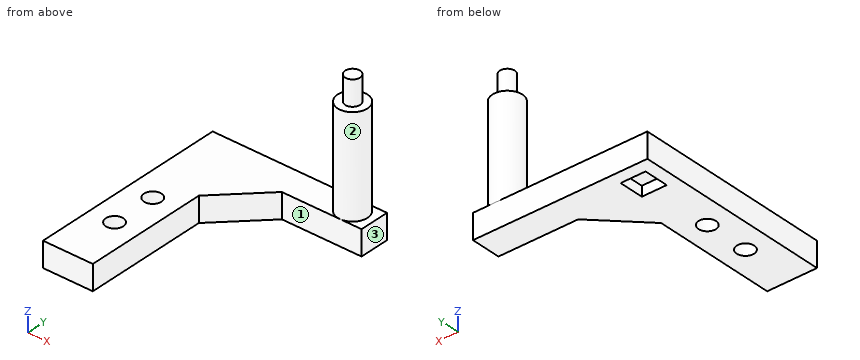
```python
from build123d import *

# Parameters (mm, degrees)
SKIZZE2_W                       = 10
SKIZZE2_H                       = 40
AUFSATZ_LINEAR_AUSTRAGEN1_DEPTH = 5
SKIZZE4_R                       = 1.75
SCHNITT_LINEAR_AUSTRAGEN1_DEPTH = 5
SKIZZE5_W                       = 5
SKIZZE5_H                       = 5
SCHNITT_LINEAR_AUSTRAGEN2_DEPTH = 2
SKIZZE6_W                       = 25
SKIZZE6_H                       = 6
AUFSATZ_LINEAR_AUSTRAGEN3_DEPTH = 5
SKIZZE7_R                       = 3
AUFSATZ_LINEAR_AUSTRAGEN4_DEPTH = 20
SKIZZE8_R                       = 1.5
AUFSATZ_LINEAR_AUSTRAGEN5_DEPTH = 5
AUFSATZ_LINEAR_AUSTRAGEN6_DEPTH = 5


with BuildPart() as part:
    # Skizze2 → Aufsatz-Linear austragen1 (new body)
    with BuildSketch(Plane.XY):
        Rectangle(SKIZZE2_W, SKIZZE2_H)
    extrude(amount=AUFSATZ_LINEAR_AUSTRAGEN1_DEPTH)

    # Skizze4 → Schnitt-Linear austragen1 (cut)
    with BuildSketch(Plane.XY.offset(5)):
        Circle(SKIZZE4_R)
        with Locations((0, -9)):
            Circle(SKIZZE4_R)
    extrude(amount=-SCHNITT_LINEAR_AUSTRAGEN1_DEPTH, mode=Mode.SUBTRACT)

    # Skizze5 → Schnitt-Linear austragen2 (cut)
    with BuildSketch(Plane(origin=(0, 0, 0), x_dir=(-1, 0, 0), z_dir=(0, 0, -1))):
        with Locations((0, 15)):
            Rectangle(SKIZZE5_W, SKIZZE5_H)
    extrude(amount=-SCHNITT_LINEAR_AUSTRAGEN2_DEPTH, mode=Mode.SUBTRACT)

    # Skizze6 → Aufsatz-Linear austragen3 (add)
    with BuildSketch(Plane.XY.offset(5)):
        with Locations((17.5, 17)):
            Rectangle(SKIZZE6_W, SKIZZE6_H)
    extrude(amount=-AUFSATZ_LINEAR_AUSTRAGEN3_DEPTH)

    # Skizze7 → Aufsatz-Linear austragen4 (add)
    with BuildSketch(Plane.XY.offset(5)):
        with Locations(Location((25.65, 17, 0), (0, 0, 270))):
            Circle(SKIZZE7_R)
    extrude(amount=AUFSATZ_LINEAR_AUSTRAGEN4_DEPTH)

    # Skizze8 → Aufsatz-Linear austragen5 (add)
    with BuildSketch(Plane.XY.offset(25)):
        with Locations((25.65, 17)):
            Circle(SKIZZE8_R)
    extrude(amount=AUFSATZ_LINEAR_AUSTRAGEN5_DEPTH)

    # Skizze9 → Aufsatz-Linear austragen6 (add)
    with BuildSketch(Plane.XY.offset(5)):
        Polygon((5, 14), (5, 10.656854249), (8.343145751, 14), align=None)
        Polygon((5, 10.656854249), (5, 5), (14, 14), (8.343145751, 14), align=None)
    extrude(amount=-AUFSATZ_LINEAR_AUSTRAGEN6_DEPTH)


solid = part.part
```
Part model, mm, in its own coordinate system. Face numbers are marked on the shaded views. A direction names the side the tool comes from. Give positions to 0.01 mm unless a question says otherwise; leave off trailing zeros. Write each loop counter-clockwise with the first axis right and the second up, starting at its lowest first coordinate (ties: lowest second). Pieces come first, ordered by that corner, then holes. Notation, with made-up numbers: (76.25, 41.5) -> (104.25, 41.5) arc R18 ccw to (104.25, 73.5) -> close; hole circle Ø7 at (10.25, 14.25). An arc over 180 degrees is marked (long way). Put each result on its own line as item: value. Start each with the question number.
Item 1: Cut at D-D (z = 20.5). List the corners of the cut face in (x, y).
Item 2: Wall check: L1, parallel to Y at x = 0, z = 3.2; L2, parallel to Y at x = 0, z = 1.25; L3, parallel to Z at x = 1.5, y = 8. Give the ranges that are in metal, low to high. Write a range as [from, to].
Item 3: Cut at A-A (y = -9). List the corners of the cut face in (x, z).
Item 4: Cut at B-B (x = 0). List the corners of the cut face in (y, z).
Item 5: Which spindle directions (+Z, -Z, +X, -X, +Y, -Y) get a long thin tool onto all of the face, cutting with end or side? Do the marked faces 1, 2 and 3. Say none if no direction does.
Item 6: Cut at C-C (y = 17). List the corners of the cut face in (x, z).
Item 7: Pin check, flat tips, straight feed: pin 1 Ø4.5 at (x, y) = (0, -9) entering from +Z; pin 2 Ø4 at (x, z) = (20, 2) entering from -Y; pin 3 Ø4 at (x, y) = (0, 15) entering from -Z; pin 4 Ø3 at (x, y) = (0, 0) entering from +Z. Stop position of each tip, or through.
Answer list:
1. outline: circle Ø6 at (25.65, 17)
2. L1: y = [-20, -10.75], [-7.25, -1.75], [1.75, 20]
2. L2: y = [-20, -10.75], [-7.25, -1.75], [1.75, 12.5], [17.5, 20]
2. L3: z = [0, 5]
3. outline: (-5, 0) -> (-1.75, 0) -> (-1.75, 5) -> (-5, 5) -> close; (1.75, 0) -> (5, 0) -> (5, 5) -> (1.75, 5) -> close
4. outline: (-20, 0) -> (-10.75, 0) -> (-10.75, 5) -> (-20, 5) -> close; (-7.25, 0) -> (-1.75, 0) -> (-1.75, 5) -> (-7.25, 5) -> close; (1.75, 0) -> (12.5, 0) -> (12.5, 2) -> (17.5, 2) -> (17.5, 0) -> (20, 0) -> (20, 5) -> (1.75, 5) -> close
5. face 1: +Z, -Z, +X, -Y
5. face 2: +Z
5. face 3: +Z, -Z, +X, +Y, -Y
6. outline: (-5, 0) -> (-2.5, 0) -> (-2.5, 2) -> (2.5, 2) -> (2.5, 0) -> (30, 0) -> (30, 5) -> (28.65, 5) -> (28.65, 25) -> (27.15, 25) -> (27.15, 30) -> (24.15, 30) -> (24.15, 25) -> (22.65, 25) -> (22.65, 5) -> (-5, 5) -> close
7. pin 1: stops at z = 5
7. pin 2: stops at y = 14
7. pin 3: stops at z = 2
7. pin 4: passes through
